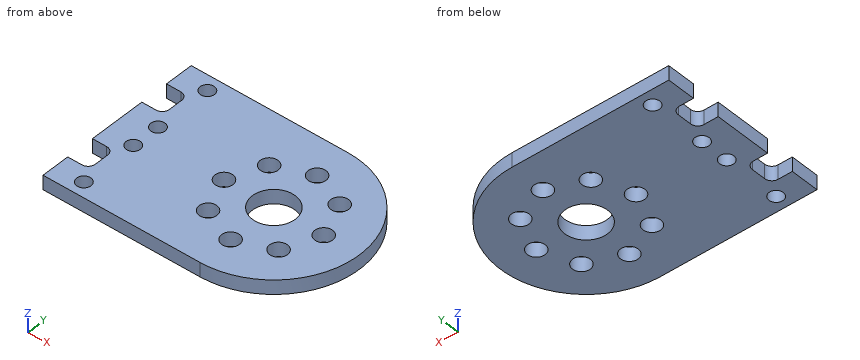
```python
from build123d import *

# Parameters (mm, degrees)
SKETCH_8_R      = 1.25
SKETCH_8_R_2    = 3
SKETCH_8_R_3    = 1
EXTRUDE_1_DEPTH = 2


with BuildPart() as part:
    # 草圖8 → 填料-伸長1 (new body)
    with BuildSketch(Plane.XY):
        with BuildLine():
            Line((-25.40478598, 11.861352689), (-25.40478598, 7.861352689))
            Line((-25.40478598, 7.861352689), (-23.40478598, 7.861352689))
            ThreePointArc((-23.40478598, 7.861352689), (-22.697679198, 7.56845947), (-22.40478598, 6.861352689))
            Line((-22.40478598, 6.861352689), (-22.40478598, 4.861352689))
            ThreePointArc((-22.40478598, 4.861352689), (-22.697679198, 4.154245908), (-23.40478598, 3.861352689))
            Line((-23.40478598, 3.861352689), (-25.40478598, 3.861352689))
            Line((-25.40478598, 3.861352689), (-25.40478598, -4.138647311))
            Line((-25.40478598, -4.138647311), (-23.40478598, -4.138647311))
            ThreePointArc((-23.40478598, -4.138647311), (-22.697679198, -4.43154053), (-22.40478598, -5.138647311))
            Line((-22.40478598, -5.138647311), (-22.40478598, -7.138647311))
            ThreePointArc((-22.40478598, -7.138647311), (-22.697679198, -7.845754092), (-23.40478598, -8.138647311))
            Line((-23.40478598, -8.138647311), (-25.40478598, -8.138647311))
            Line((-25.40478598, -8.138647311), (-25.40478598, -12.138647311))
            Line((-25.40478598, -12.138647311), (-3.40478598, -12.138647311))
            ThreePointArc((-3.40478598, -12.138647311), (8.59521402, -0.138647311), (-3.40478598, 11.861352689))
            Line((-3.40478598, 11.861352689), (-25.40478598, 11.861352689))
        make_face()
        with Locations((-3.40478598, 6.861352689)):
            Circle(SKETCH_8_R, mode=Mode.SUBTRACT)
        with Locations((1.544961489, 4.811100157)):
            Circle(SKETCH_8_R, mode=Mode.SUBTRACT)
        with Locations((-3.40478598, -0.138647311)):
            Circle(SKETCH_8_R_2, mode=Mode.SUBTRACT)
        with Locations((3.59521402, -0.138647311)):
            Circle(SKETCH_8_R, mode=Mode.SUBTRACT)
        with Locations((1.544961489, -5.08839478)):
            Circle(SKETCH_8_R, mode=Mode.SUBTRACT)
        with Locations((-3.40478598, -7.138647311)):
            Circle(SKETCH_8_R, mode=Mode.SUBTRACT)
        with Locations((-8.354533448, -5.08839478)):
            Circle(SKETCH_8_R, mode=Mode.SUBTRACT)
        with Locations((-10.40478598, -0.138647311)):
            Circle(SKETCH_8_R, mode=Mode.SUBTRACT)
        with Locations((-8.354533448, 4.811100157)):
            Circle(SKETCH_8_R, mode=Mode.SUBTRACT)
        with Locations((-21.40478598, 9.861352689)):
            Circle(SKETCH_8_R_3, mode=Mode.SUBTRACT)
        with Locations((-21.40478598, 1.861352689)):
            Circle(SKETCH_8_R_3, mode=Mode.SUBTRACT)
        with Locations((-21.40478598, -2.138647311)):
            Circle(SKETCH_8_R_3, mode=Mode.SUBTRACT)
        with Locations((-21.40478598, -10.138647311)):
            Circle(SKETCH_8_R_3, mode=Mode.SUBTRACT)
    extrude(amount=EXTRUDE_1_DEPTH)


solid = part.part
```
For this review, take the finished solid that the model builds, in its own axes (mm). Give positions to 0.01 mm unless a question says otherwise; leave off trailing zeros. Loops run counter-clockwise (first coordinate to the right, second up) from the corner with the lowest first, then second, coordinate; pieces in that order, holes last. Notation, with made-up numbers: M -0.5,-18.5 L 47.5,-18.5 A25 cw 47.5,-0.5 Z; hole C 32.5,-37 d1. An arc over 180 degrees is marked long. One line per item, written item: value. Start each with the question number.
Q1. Add section C-C (x = 1). Give the boundary of the cut face in (y, z).
Q2. Add section A-A (x = -21). Give the boundary of the cut face in (y, z), and give its area (3 significant figures).
Q3. For L1, parallel to Y at x = -3.5, z = 1.7; L2, parallel to Y at x = -21.5, z = 0.2; L3, parallel to Y at x = -21, z = 1.4, list the stretches that pass through material, from the lowest coordinate up.
Q4. Clearance check with flat-ended pins moving along their axes: pin 1 Ø2 at (x, y) = (1.54, 4.81) entering from -Z; pin 2 Ø1 at (y, z) = (5.5, 0.5) entering from -X. State where each tip first meets the part, or that it passes through.
Q5. Add section D-D (y = 4.25). Give the boundary of the cut face in (x, z).
Q6. Add section B-B (y = -7.5). Give the boundary of the cut face in (x, z).
Reply:
1. outline: M -11.3,0 L -6.21,0 L -6.21,2 L -11.3,2 Z; M -3.96,0 L 3.69,0 L 3.69,2 L -3.96,2 Z; M 5.94,0 L 11.02,0 L 11.02,2 L 5.94,2 Z
2. outline: M -12.14,0 L -11.05,0 L -11.05,2 L -12.14,2 Z; M -9.22,0 L -3.05,0 L -3.05,2 L -9.22,2 Z; M -1.22,0 L 0.95,0 L 0.95,2 L -1.22,2 Z; M 2.78,0 L 8.95,0 L 8.95,2 L 2.78,2 Z; M 10.78,0 L 11.86,0 L 11.86,2 L 10.78,2 Z
2. area: 33.4 mm²
3. L1: -12.14 to -8.39, -5.89 to -3.14, 2.86 to 5.61, 8.11 to 11.86
3. L2: -12.14 to -11.13, -9.14 to -3.13, -1.14 to 0.87, 2.86 to 8.87, 10.86 to 11.86
3. L3: -12.14 to -11.05, -9.22 to -3.05, -1.22 to 0.95, 2.78 to 8.95, 10.78 to 11.86
4. pin 1: through
4. pin 2: x = -22.4
5. outline: M -22.61,0 L -9.47,0 L -9.47,2 L -22.61,2 Z; M -7.24,0 L 0.43,0 L 0.43,2 L -7.24,2 Z; M 2.66,0 L 7.76,0 L 7.76,2 L 2.66,2 Z
6. outline: M -22.47,0 L -4.6,0 L -4.6,2 L -22.47,2 Z; M -2.21,0 L 6.07,0 L 6.07,2 L -2.21,2 Z
